from build123d import *

# Parameters (mm, degrees)
SKETCH1_W            = 45.5
SKETCH1_H            = 18
BOSS_EXTRUDE1_DEPTH  = 3
SKETCH2_W            = 3
SKETCH2_H            = 18
SKETCH2_W_2          = 1.5
BOSS_EXTRUDE2_DEPTH  = 20
SKETCH6_W            = 2
SKETCH6_H            = 20
BOSS_EXTRUDE5_DEPTH  = 5
SKETCH7_R            = 2
CUT_EXTRUDE2_DEPTH   = 2
BOSS_EXTRUDE9_DEPTH  = 75.5
SKETCH9_W            = 18
SKETCH9_H            = 3
BOSS_EXTRUDE10_DEPTH = 40


with BuildPart() as part:
    # Sketch1 → Boss-Extrude1 (new body)
    with BuildSketch(Plane(origin=(0, 0, 0), x_dir=(1, 0, 0), z_dir=(0, 1, 0))):
        Rectangle(SKETCH1_W, SKETCH1_H)
    extrude(amount=BOSS_EXTRUDE1_DEPTH)

    # Sketch2 → Boss-Extrude2 (add)
    with BuildSketch(Plane(origin=(0, 3, 0), x_dir=(1, 0, 0), z_dir=(0, 1, 0))):
        with Locations((-21.25, 0)):
            Rectangle(SKETCH2_W, SKETCH2_H)
        with Locations((22, 0)):
            Rectangle(SKETCH2_W_2, SKETCH2_H)
    extrude(amount=BOSS_EXTRUDE2_DEPTH)

    # Sketch6 → Boss-Extrude5 (add)
    with BuildSketch(Plane(origin=(22.75, 0, 0), x_dir=(0, 0, -1), z_dir=(1, 0, 0))):
        with Locations((-8, 13)):
            Rectangle(SKETCH6_W, SKETCH6_H)
    extrude(amount=BOSS_EXTRUDE5_DEPTH)

    # Sketch7 → Cut-Extrude2 (cut)
    with BuildSketch(Plane.XY.offset(9)):
        with Locations((25.05, 8)):
            Circle(SKETCH7_R)
        with Locations((25.05, 18)):
            Circle(SKETCH7_R)
    extrude(amount=-CUT_EXTRUDE2_DEPTH, mode=Mode.SUBTRACT)

    # 3DSketch1 → Boss-Extrude9 (add)
    with BuildSketch(Plane(origin=(-22.75, 0, 9), x_dir=(0, -0.3396444637775567, -0.9405538996916956), z_dir=(-1, 0, 0))):
        with BuildLine():
            Line((0, 0), (2.207689015, 6.113600348))
            Line((2.207689015, 6.113600348), (4.696214266, 5.214966229))
            ThreePointArc((4.696214266, 5.214966229), (8.301670881, -2.466223951), (15.982861062, 1.139232664))
            Line((15.982861062, 1.139232664), (19.137659209, 0))
            Line((19.137659209, 0), (16.929970194, -6.113600348))
            Line((16.929970194, -6.113600348), (0, 0))
        make_face()
    extrude(amount=-BOSS_EXTRUDE9_DEPTH)

    # Sketch9 → Boss-Extrude10 (add)
    with BuildSketch(Plane(origin=(22.75, 0, 0), x_dir=(0, 0, -1), z_dir=(1, 0, 0))):
        with Locations((0, 1.5)):
            Rectangle(SKETCH9_W, SKETCH9_H)
    extrude(amount=BOSS_EXTRUDE10_DEPTH)


solid = part.part
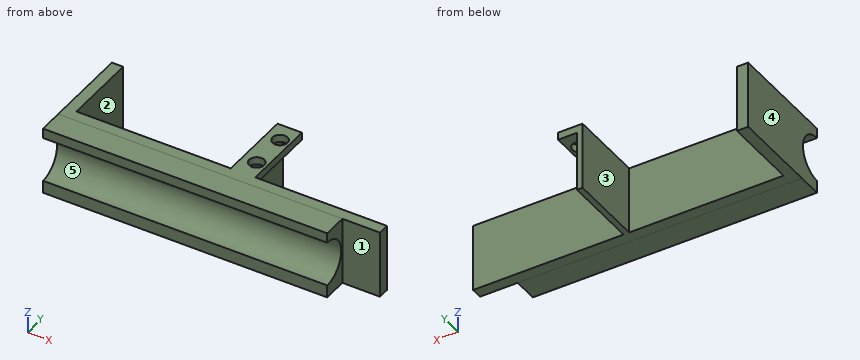
For this review, take the finished solid that the model builds, in its own axes (mm). Face numbers are marked on the shaded views. A direction names the side the tool comes from. Round coordinates to 2 decimals unless told otherwise and drop trailing zeros. Loops run counter-clockwise (first coordinate to the right, second up) from the corner with the lowest first, then second, coordinate; pieces in that order, holes last. Notation, with made-up numbers: (-22, 55.5) - (-4, 55.5) arc R8 cw to (-4, 63.5) - close; hole circle Ø4 at (72.25, 75). An arc over 180 degrees is marked (long way). Answer as CSV lines item,"result".
(1) Consider section B-B on x = 25.05. Give the boundary of the cut face in (y, z), then the cut area to 3 significant figures.
Checked values:
outline,"(-6.5, -9) - (3, -9) - (3, 7) - (6, 7) - (6, 9) - (-6.5, 9) - (-6.5, 6.35) arc R6 cw to (-6.5, -5.65) - close; (10, 7) - (16, 7) - (16, 9) - (10, 9) - close; (20, 7) - (23, 7) - (23, 9) - (20, 9) - close"
area,"138 mm2"
(2) Wall thickness on line 1 (Y direction, x = 25.05, z = 8.05); line 2 (X direction, y = 12, z = -0.75); line 3 (X direction, y = -5, z = -6): over which ranges is each line inside the solid? List them lowest first.
Checked values:
line 1,"y = -6.5 to 6, 10 to 16, 20 to 23"
line 2,"x = -22.75 to -19.75, 21.25 to 22.75"
line 3,"x = -22.75 to 52.75"
(3) Consider section A-A on y = 18. Give the boundary of the cut face in (x, z), then the cut area to 3 significant figures.
Checked values:
outline,"(-22.75, -9) - (-19.75, -9) - (-19.75, 9) - (-22.75, 9) - close; (21.25, -9) - (22.75, -9) - (22.75, 7) - (23.05, 7) - (23.05, 9) - (21.25, 9) - close; (27.05, 7) - (27.75, 7) - (27.75, 9) - (27.05, 9) - close"
area,"83.0 mm2"
(4) Tool access review of the marked faces 1 and 2: name each direction out of +Z, -Z, +X, -X, +Y, -Y from which nothing blocks a thin tool from reaching the whole face with its end or side.
Checked values:
face 1,"+Z, -Z, +X, -Y"
face 2,"+Z, -Z, +Y"
(5) Consider section C-C on z = -4.75. Give the boundary of the cut face in (x, y).
Checked values:
outline,"(-22.75, -3.35) - (52.75, -3.35) - (52.75, 0) - (62.75, 0) - (62.75, 3) - (22.75, 3) - (22.75, 23) - (21.25, 23) - (21.25, 3) - (-19.75, 3) - (-19.75, 23) - (-22.75, 23) - close"
(6) Mouldability with a two-part tool opening along X and no side actions: class the marked faces 3, 4 and 5 as +X half, -X half, draft (parallel to the pull), parting line (faces both ways), or undercut.
Checked values:
face 3,"undercut"
face 4,"-X half"
face 5,"draft"
(7) Consider section D-D on x = 43.5. Give the boundary of the cut face in (y, z).
Checked values:
outline,"(-6.5, -9) - (3, -9) - (3, 9) - (-6.5, 9) - (-6.5, 6.35) arc R6 cw to (-6.5, -5.65) - close"
(8) Insertion check: P1, Ø3, axis at x = 37, z = 4, coming from the +Y side; P2, Ø9, axis at y = 11, z = 3, coming from the +X side; P3, Ø2.5, axis at x = 26, y = 15, coming from the -Z side. Each pin has a flat end and moves straight along its axis. Give the tip position at first contact, or say it passes through.
Checked values:
P1,"stops at y = 3"
P2,"stops at x = 27.75"
P3,"stops at z = 7"
